```python
from build123d import *

# Parameters (mm, degrees)
BOSS_EXTRUDE1_DEPTH                                  = 300
SKETCH2_R                                            = 22.5
CUT_EXTRUDE1_DEPTH                                   = 319.198051534
SKETCH3_W                                            = 40
SKETCH3_H                                            = 56
CUT_EXTRUDE2_DEPTH                                   = 10
SKETCH4_W                                            = 40
SKETCH4_H                                            = 41
CUT_EXTRUDE3_DEPTH                                   = 10
FILLET1_R                                            = 3
CSK_FOR_M10_COUNTERSUNK_FLAT_HEAD_SCREW1_D           = 11
CSK_FOR_M10_COUNTERSUNK_FLAT_HEAD_SCREW1_DEPTH       = 20.003
CSK_FOR_M10_COUNTERSUNK_FLAT_HEAD_SCREW1_CSINK_D     = 20
CSK_FOR_M10_COUNTERSUNK_FLAT_HEAD_SCREW1_CSINK_ANGLE = 90
CSK_FOR_M10_COUNTERSUNK_FLAT_HEAD_SCREW1_TIP         = 3.304733405


with BuildPart() as part:
    # Sketch1 → Boss-Extrude1 (new body)
    with BuildSketch(Plane.XY):
        Polygon((0, -37.5), (0, 37.5), (75, 37.5), (75, 31.15), (6.35, 31.15), (6.35, -31.15), (75, -31.15), (75, -37.5), align=None)
    extrude(amount=BOSS_EXTRUDE1_DEPTH)

    # Sketch2 → Cut-Extrude1 (cut, through all)
    with BuildSketch(Plane(origin=(0, 37.5, 0), x_dir=(1, 0, 0), z_dir=(0, 1, 0))):
        with Locations(Location((40, -150, 0), (0, 0, 270))):
            Circle(SKETCH2_R)
    extrude(amount=-CUT_EXTRUDE1_DEPTH, mode=Mode.SUBTRACT)

    # Sketch3 → Cut-Extrude2 (cut)
    with BuildSketch(Plane.XZ.offset(37.5)):
        with Locations((40, 63)):
            Rectangle(SKETCH3_W, SKETCH3_H)
    extrude(amount=-CUT_EXTRUDE2_DEPTH, mode=Mode.SUBTRACT)

    # Sketch4 → Cut-Extrude3 (cut)
    with BuildSketch(Plane(origin=(0, 37.5, 0), x_dir=(1, 0, 0), z_dir=(0, 1, 0))):
        with Locations((40, -84.5)):
            Rectangle(SKETCH4_W, SKETCH4_H)
    extrude(amount=-CUT_EXTRUDE3_DEPTH, mode=Mode.SUBTRACT)

    # Fillet1
    fillet1_edges = [part.edges().sort_by_distance(p)[0] for p in [
        (20, -34.325, 91),
        (60, -34.325, 91),
        (60, -34.325, 35),
        (20, -34.325, 35),
        (60, 34.325, 105),
        (20, 34.325, 105),
        (20, 34.325, 64),
        (60, 34.325, 64),
    ]]
    fillet(fillet1_edges, radius=FILLET1_R)

    # CSK for M10 Countersunk Flat Head Screw1
    with Locations(Plane.ZY):
        with Locations((74.704121605, 4.01110333)):
            CounterSinkHole(CSK_FOR_M10_COUNTERSUNK_FLAT_HEAD_SCREW1_D / 2, CSK_FOR_M10_COUNTERSUNK_FLAT_HEAD_SCREW1_CSINK_D / 2, depth=CSK_FOR_M10_COUNTERSUNK_FLAT_HEAD_SCREW1_DEPTH, counter_sink_angle=CSK_FOR_M10_COUNTERSUNK_FLAT_HEAD_SCREW1_CSINK_ANGLE)
            with Locations((0, 0, -(CSK_FOR_M10_COUNTERSUNK_FLAT_HEAD_SCREW1_DEPTH + CSK_FOR_M10_COUNTERSUNK_FLAT_HEAD_SCREW1_TIP / 2))):  # 118° drill point
                Cone(0, CSK_FOR_M10_COUNTERSUNK_FLAT_HEAD_SCREW1_D / 2, CSK_FOR_M10_COUNTERSUNK_FLAT_HEAD_SCREW1_TIP, mode=Mode.SUBTRACT)


solid = part.part
```
Work out the finished part from the listing and answer in its coordinate system (mm). A direction names the side the tool comes from. Round coordinates to 2 decimals unless told otherwise and drop trailing zeros. Write each loop counter-clockwise with the first axis right and the second up, starting at its lowest first coordinate (ties: lowest second). Pieces come first, ordered by that corner, then holes. Notation, with made-up numbers: (-36.5, 87.25) -> (-8.5, 87.25) arc R29 ccw to (-8.5, 121.25) -> close; hole circle Ø3 at (0.25, 51.25). An arc over 180 degrees is marked (long way). Write each question's results on one line, items separated by ' | '.
1) The part is cut by section B-B (z = 150). Write down the section's boundary in (x, y), and give its area (3 significant figures).
Findings:
outline: (0, -37.5) -> (17.5, -37.5) -> (17.5, -31.15) -> (6.35, -31.15) -> (6.35, 31.15) -> (17.5, 31.15) -> (17.5, 37.5) -> (0, 37.5) -> close; (62.5, -37.5) -> (75, -37.5) -> (75, -31.15) -> (62.5, -31.15) -> close; (62.5, 31.15) -> (75, 31.15) -> (75, 37.5) -> (62.5, 37.5) -> close | area: 777 mm²
2) Which of the six approach directions +Z, -Z, +X, -X, +Y, -Y give full straight-line access (tool end or side, diameter ignored) to faces 1 (the flat face through (20, 34, 85)), 2 (the flat face through (40, -31.15, 181)), 3 (the flat face through (40, -34, 35)), 4 (the cylindrical face through (5.44, 4.25, 80.2)), 5 (the flat face through (40, 34, 64))?
Findings:
face 1: +Y | face 2: +Z, -Z, +X | face 3: -Y | face 4: +X, -X | face 5: +Y, -Y
3) The part is cut by section C-C (z = 250). Write down the section's boundary in (x, y).
Findings:
outline: (0, -37.5) -> (75, -37.5) -> (75, -31.15) -> (6.35, -31.15) -> (6.35, 31.15) -> (75, 31.15) -> (75, 37.5) -> (0, 37.5) -> close
4) Flat-ended cylindrical pins translate along their axes: pin 1 (6 mm diameter, centred on y = 21, z = 117.5, fed in from +X); pin 2 (12.5 mm diameter, centred on y = 4.01, z = 74.7, fed in from -X); pin 3 (10 mm diameter, centred on x = 14.5, y = -19.5, fed in from +Z). Find the tip coordinate at first contact, or state that the pin passes through.
Findings:
pin 1: stops at x = 6.35 | pin 2: stops at x = 3.75 | pin 3: passes through
5) The part is cut by section A-A (x = 40). Write down the section's boundary in (y, z).
Findings:
outline: (-37.5, 0) -> (-31.15, 0) -> (-31.15, 35) -> (-37.5, 35) -> close; (-37.5, 91) -> (-31.15, 91) -> (-31.15, 127.5) -> (-37.5, 127.5) -> close; (-37.5, 172.5) -> (-31.15, 172.5) -> (-31.15, 300) -> (-37.5, 300) -> close; (31.15, 0) -> (37.5, 0) -> (37.5, 64) -> (31.15, 64) -> close; (31.15, 105) -> (37.5, 105) -> (37.5, 127.5) -> (31.15, 127.5) -> close; (31.15, 172.5) -> (37.5, 172.5) -> (37.5, 300) -> (31.15, 300) -> close
6) For a pull along Z with two mould halves and no side action, classify faces 6 (the flat face through (4, -5, 0)), 7 (the flat face through (60, 34, 85)), 8 (the flat face through (6.35, 0, 148)) as +Z half, -Z half, draft (parallel to the pull), parting line (faces both ways), or undercut.
Findings:
face 6: -Z half | face 7: undercut | face 8: draft
7) Consider line 1 along Y through (x, z) = (48, 273); line 2 along X through (y, z) = (-34.5, 150); line 3 along Z through (x, y) = (31.5, -32.5). Determine where each line is inside the solid, lowest interval first. Write a range as [from, to].
Findings:
line 1: y = [-37.5, -31.15], [31.15, 37.5] | line 2: x = [0, 17.5], [62.5, 75] | line 3: z = [0, 35], [91, 129.17], [170.83, 300]
8) The part is cut by section D-D (y = 17). Write down the section's boundary in (x, z).
Findings:
outline: (0, 0) -> (6.35, 0) -> (6.35, 300) -> (0, 300) -> close
